from build123d import *

# Parameters (mm, degrees)
SKETCH1_R           = 6
SKETCH1_R_2         = 1.1
BOSS_EXTRUDE1_DEPTH = 3.9
SKETCH5_R           = 8
SKETCH5_R_2         = 2.05
SKETCH5_R_3         = 0.525
BOSS_EXTRUDE3_DEPTH = 0.5
BOSS_EXTRUDE4_DEPTH = 6.5


with BuildPart() as part:
    # Sketch1 → Boss-Extrude1 (new body)
    with BuildSketch(Plane.XY):
        with BuildLine():
            Line((-2.5, -27.5), (2.5, -27.5))
            Line((2.5, -27.5), (2.5, -12.951833847))
            ThreePointArc((2.5, -12.951833847), (3.295532486, -9.043154047), (5.555555556, -5.756370599))
            ThreePointArc((5.555555556, -5.756370599), (0, 8), (-5.555555556, -5.756370599))
            ThreePointArc((-5.555555556, -5.756370599), (-3.295532486, -9.043154047), (-2.5, -12.951833847))
            Line((-2.5, -12.951833847), (-2.5, -27.5))
        make_face()
        Circle(SKETCH1_R, mode=Mode.SUBTRACT)
        with Locations((0, -23.5)):
            Circle(SKETCH1_R_2, mode=Mode.SUBTRACT)
    extrude(amount=BOSS_EXTRUDE1_DEPTH)

    # Sketch5 → Boss-Extrude3 (add)
    with BuildSketch(Plane(origin=(0, 0, 0), x_dir=(-1, 0, 0), z_dir=(0, 0, -1))):
        Circle(SKETCH5_R)
        Circle(SKETCH5_R_2, mode=Mode.SUBTRACT)
        with Locations((4.2, 0)):
            Circle(SKETCH5_R_3, mode=Mode.SUBTRACT)
        with Locations((-4.2, 0)):
            Circle(SKETCH5_R_3, mode=Mode.SUBTRACT)
    extrude(amount=-BOSS_EXTRUDE3_DEPTH)

    # Sketch7 → Boss-Extrude4 (add)
    with BuildSketch(Plane.XZ.offset(27.5)):
        with BuildLine():
            ThreePointArc((7, 7.666888651), (4.877255668, 5.281037947), (1.997835367, 3.9))
            Line((1.997835367, 3.9), (2.5, 3.9))
            Line((2.5, 3.9), (2.5, 0))
            ThreePointArc((2.5, 0), (6.103916398, 3.038777275), (7, 7.666888651))
        make_face()
        with BuildLine():
            Line((-2.5, 3.9), (-1.997835367, 3.9))
            ThreePointArc((-1.997835367, 3.9), (-4.877255668, 5.281037947), (-7, 7.666888651))
            ThreePointArc((-7, 7.666888651), (-6.103916398, 3.038777275), (-2.5, 0))
            Line((-2.5, 0), (-2.5, 3.9))
        make_face()
    extrude(amount=-BOSS_EXTRUDE4_DEPTH)


solid = part.part
Part model, mm, in its own coordinate system. A direction names the side the tool comes from. Give positions to 0.01 mm unless a question says otherwise; leave off trailing zeros. Loops run counter-clockwise (first coordinate to the right, second up) from the corner with the lowest first, then second, coordinate; pieces in that order, holes last.
(1) Band-saw the part on A-A (x = 0). Write the cut outline in (y, z).
Return value:
outline: (-27.5, 0) - (-24.6, 0) - (-24.6, 3.9) - (-27.5, 3.9) - close; (-22.4, 0) - (-2.05, 0) - (-2.05, 0.5) - (-6, 0.5) - (-6, 3.9) - (-22.4, 3.9) - close; (2.05, 0) - (8, 0) - (8, 3.9) - (6, 3.9) - (6, 0.5) - (2.05, 0.5) - close
(2) Band-saw the part on D-D (y = -23.5). Write the cut outline in (x, z).
Return value:
outline: (-7, 7.67) arc R7.08 ccw to (-2.5, 0) - (-1.1, 0) - (-1.1, 3.9) - (-2, 3.9) arc R8.11 cw to start; (1.1, 0) - (2.5, 0) arc R7.08 ccw to (7, 7.67) arc R8.11 cw to (2, 3.9) - (1.1, 3.9) - close
(3) 3-axis set-ups, long thin cutter, end or side, ignore diameter. For faces 1 (the cylindrical face through (4.9, -24.3, 5.3)), 2 (the cylindrical face through (-6, 0, 2)), 3 (the flat face through (2.5, -17, 2)): which of +Z, -Z, +X, -X, +Y, -Y reach the whole face in a straight line?
Return value:
face 1: +Z, +Y, -Y
face 2: +Z
face 3: +Z, -Z, +X
(4) Drill centre lines: line 1 along Y through (x, z) = (0, 1); line 2 along Z through (x, y) = (-0.25, -9.5); line 3 along Y through (x, z) = (5.75, 6). Where is each one in solid material? Low to high.
Return value:
line 1: y = -27.5 to -24.6, -22.4 to -6, 6 to 8
line 2: z = 0 to 3.9
line 3: y = -27.5 to -21
(5) Band-saw the part on C-C (z = 4.75). Write the cut outline in (x, y).
Return value:
outline: (-6.83, -27.5) - (-4.08, -27.5) - (-4.08, -21) - (-6.83, -21) - close; (4.08, -27.5) - (6.83, -27.5) - (6.83, -21) - (4.08, -21) - close
(6) Band-saw the part on B-B (y = 0). Write the cut outline in (x, z) (3 decimals).
Return value:
outline: (-8, 0) - (-4.725, 0) - (-4.725, 0.5) - (-6, 0.5) - (-6, 3.9) - (-8, 3.9) - close; (-3.675, 0) - (-2.05, 0) - (-2.05, 0.5) - (-3.675, 0.5) - close; (2.05, 0) - (3.675, 0) - (3.675, 0.5) - (2.05, 0.5) - close; (4.725, 0) - (8, 0) - (8, 3.9) - (6, 3.9) - (6, 0.5) - (4.725, 0.5) - close
(7) Pin check, flat tips, straight feed: pin 1 (3.5 mm diameter, centred on x = 0, y = -23.5, fed in from +Z); pin 2 (1.5 mm diameter, centred on y = -10.5, z = 1, fed in from -X); pin 3 (2.5 mm diameter, centred on x = -3.5, z = 4.5, fed in from +Y). Stop position of each tip, or through.
Return value:
pin 1: stops at z = 3.9
pin 2: stops at x = -3.03
pin 3: stops at y = 7.63
